from build123d import *

# Parameters (mm, degrees)
BOSS_EXTRUDE1_DEPTH = 5
CUT_EXTRUDE1_DEPTH  = 12
BOSS_EXTRUDE2_DEPTH = 10
FILLET1_R           = 0.5
BOSS_EXTRUDE3_START = -5
SKETCH4_R           = 3.6
BOSS_EXTRUDE3_DEPTH = 6
SKETCH6_R           = 1.6
CUT_EXTRUDE2_DEPTH  = 63.825154198
CUT_EXTRUDE3_DEPTH  = 6


with BuildPart() as part:
    # Sketch1 → Boss-Extrude1 (new body)
    with BuildSketch(Plane(origin=(0, 0, 0), x_dir=(1, 0, 0), z_dir=(0, 1, 0))):
        with BuildLine():
            Line((-44, -35), (44, -35))
            ThreePointArc((44, -35), (48.949747468, -32.949747468), (51, -28))
            Line((51, -28), (51, 28))
            ThreePointArc((51, 28), (48.949747468, 32.949747468), (44, 35))
            Line((44, 35), (-44, 35))
            ThreePointArc((-44, 35), (-48.949747468, 32.949747468), (-51, 28))
            Line((-51, 28), (-51, -28))
            ThreePointArc((-51, -28), (-48.949747468, -32.949747468), (-44, -35))
        make_face()
    extrude(amount=BOSS_EXTRUDE1_DEPTH)

    # Sketch2 → Cut-Extrude1 (cut)
    with BuildSketch(Plane(origin=(0, 5, 0), x_dir=(1, 0, 0), z_dir=(0, 1, 0))):
        with BuildLine():
            Line((-11, -29), (11, -29))
            ThreePointArc((11, -29), (12.5, -30.5), (11, -32))
            Line((11, -32), (-11, -32))
            ThreePointArc((-11, -32), (-12.5, -30.5), (-11, -29))
        make_face()
        with BuildLine():
            Line((-11, 29), (11, 29))
            ThreePointArc((11, 29), (12.5, 30.5), (11, 32))
            Line((11, 32), (-11, 32))
            ThreePointArc((-11, 32), (-12.5, 30.5), (-11, 29))
        make_face()
        with BuildLine():
            Line((-20, 6), (-20, -6))
            ThreePointArc((-20, -6), (-21.5, -7.5), (-23, -6))
            Line((-23, -6), (-23, 6))
            ThreePointArc((-23, 6), (-21.5, 7.5), (-20, 6))
        make_face()
        with BuildLine():
            Line((-10, 6), (-10, -6))
            ThreePointArc((-10, -6), (-11.5, -7.5), (-13, -6))
            Line((-13, -6), (-13, 6))
            ThreePointArc((-13, 6), (-11.5, 7.5), (-10, 6))
        make_face()
        with BuildLine():
            Line((10, 6), (10, -6))
            ThreePointArc((10, -6), (11.5, -7.5), (13, -6))
            Line((13, -6), (13, 6))
            ThreePointArc((13, 6), (11.5, 7.5), (10, 6))
        make_face()
        with BuildLine():
            Line((20, 6), (20, -6))
            ThreePointArc((20, -6), (21.5, -7.5), (23, -6))
            Line((23, -6), (23, 6))
            ThreePointArc((23, 6), (21.5, 7.5), (20, 6))
        make_face()
    extrude(amount=-CUT_EXTRUDE1_DEPTH, mode=Mode.SUBTRACT)

    # Sketch3 → Boss-Extrude2 (add)
    with BuildSketch(Plane(origin=(0, 5, 0), x_dir=(1, 0, 0), z_dir=(0, 1, 0))):
        with BuildLine():
            ThreePointArc((-44.902157539, 17.733333333), (-47, 0), (-44.902157539, -17.733333333))
            ThreePointArc((-44.902157539, -17.733333333), (-43.696427396, -18.47239681), (-42.957363919, -17.266666667))
            ThreePointArc((-42.957363919, -17.266666667), (-45, 0), (-42.957363919, 17.266666667))
            ThreePointArc((-42.957363919, 17.266666667), (-43.696427396, 18.47239681), (-44.902157539, 17.733333333))
        make_face()
        with BuildLine():
            ThreePointArc((43.957363919, 17.266666667), (46, 0), (43.957363919, -17.266666667))
            ThreePointArc((43.957363919, -17.266666667), (44.696427396, -18.47239681), (45.902157539, -17.733333333))
            ThreePointArc((45.902157539, -17.733333333), (48, 0), (45.902157539, 17.733333333))
            ThreePointArc((45.902157539, 17.733333333), (44.696427396, 18.47239681), (43.957363919, 17.266666667))
        make_face()
    extrude(amount=BOSS_EXTRUDE2_DEPTH)

    # Fillet1
    fillet1_edges = [part.edges().sort_by_distance(p)[0] for p in [
        (0, 0, -29),
        (12.5, 0, -30.5),
        (0, 0, -32),
        (-12.5, 0, -30.5),
        (0, 0, 32),
        (12.5, 0, 30.5),
        (0, 0, 29),
        (-12.5, 0, 30.5),
        (-12.5, 5, 30.5),
        (0, 5, 32),
        (12.5, 5, 30.5),
        (0, 5, 29),
        (-12.5, 5, -30.5),
        (0, 5, -29),
        (12.5, 5, -30.5),
        (0, 5, -32),
    ]]
    fillet(fillet1_edges, radius=FILLET1_R)

    # Sketch4 → Boss-Extrude3 (add)
    with BuildSketch(Plane(origin=(0, 5, 0), x_dir=(1, 0, 0), z_dir=(0, 1, 0)).offset(BOSS_EXTRUDE3_START)):
        with Locations(Location((-44, 28, 0), (0, 0, 90))):
            Circle(SKETCH4_R)
        with Locations(Location((-44, -28, 0), (0, 0, 90))):
            Circle(SKETCH4_R)
        with Locations(Location((44, -28, 0), (0, 0, 90))):
            Circle(SKETCH4_R)
        with Locations(Location((44, 28, 0), (0, 0, 90))):
            Circle(SKETCH4_R)
    extrude(amount=-BOSS_EXTRUDE3_DEPTH)

    # Sketch6 → Cut-Extrude2 (cut, through all)
    with BuildSketch(Plane(origin=(0, 5, 0), x_dir=(1, 0, 0), z_dir=(0, 1, 0))):
        with Locations(Location((-44, 28, 0), (0, 0, 270))):
            Circle(SKETCH6_R)
        with Locations(Location((44, 28, 0), (0, 0, 270))):
            Circle(SKETCH6_R)
        with Locations(Location((44, -28, 0), (0, 0, 90))):
            Circle(SKETCH6_R)
        with Locations(Location((-44, -28, 0), (0, 0, 90))):
            Circle(SKETCH6_R)
    extrude(amount=-CUT_EXTRUDE2_DEPTH, mode=Mode.SUBTRACT)

    # Sketch7 → Cut-Extrude3 (cut)
    with BuildSketch(Plane(origin=(0, 5, 0), x_dir=(1, 0, 0), z_dir=(0, 1, 0))):
        Polygon((-42.41228676, 30.75), (-45.58771324, 30.75), (-47.175426481, 28), (-45.58771324, 25.25), (-42.41228676, 25.25), (-40.824573519, 28), align=None)
        Polygon((40.824573519, 28), (42.41228676, 30.75), (45.58771324, 30.75), (47.175426481, 28), (45.58771324, 25.25), (42.41228676, 25.25), align=None)
        Polygon((42.41228676, -30.75), (45.58771324, -30.75), (47.175426481, -28), (45.58771324, -25.25), (42.41228676, -25.25), (40.824573519, -28), align=None)
        Polygon((-40.824573519, -28), (-42.41228676, -30.75), (-45.58771324, -30.75), (-47.175426481, -28), (-45.58771324, -25.25), (-42.41228676, -25.25), align=None)
    extrude(amount=-CUT_EXTRUDE3_DEPTH, mode=Mode.SUBTRACT)


solid = part.part
The listing builds one solid part. Answer for the finished solid, in the listing's coordinates (mm). A direction names the side the tool comes from. Coordinates: 2 decimals unless noted, no trailing zeros. Write each loop counter-clockwise with the first axis right and the second up, starting at its lowest first coordinate (ties: lowest second). Pieces come first, ordered by that corner, then holes. Notation, with made-up numbers: M 61.5,22.25 L 90.5,22.25 A29 ccw 90.5,59.25 Z; hole C 46,14 d5. An arc over 180 degrees is marked long. Put each result on its own line as item: value. Start each with the question number.
1. Which of the six approach directions +Z, -Z, +X, -X, +Y, -Y give full straight-line access (tool end or side, diameter ignored) to faces 1 (the flat face through (-45.4, -1, 29.2)), 2 (the cylindrical face through (21.5, 2.5, 7.5))?
2. For a pull along X with two mould halves and no side action, classify faces 3 (the flat face through (-42.6, -1, -26.8)), 4 (the cylindrical face through (-47, 10, 0)), 5 (the cylindrical face through (48.9, 2.5, 33)), 6 (the flat face through (-23, 3, 0)) as pulls with the +X half, pulls with the -X half, needs draft (parallel to the pull), parting line crosses it, or undercut.
3. Consider line 1 (Z direction, x = -9.5, y = 3.5); line 2 (X direction, y = -3.8, z = -28); line 3 (Y direction, x = -7.5, z = 20). Determine where each line is inside the solid, lowest interval first. Write a range as from..to.
4. A cutting plane is placed at D-D on z = 1. Write down the section's boundary in (x, y), then the cut area to 3 significant figures.
5. A cutting plane is placed at C-C on x = -5. Write down the section's boundary in (y, z).
6. A cutting plane is placed at A-A on x = -21.5. Write down the section's boundary in (y, z), then the cut area to 3 significant figures.
7. A cutting plane is placed at B-B on y = 8.25. Write down the section's boundary in (x, z).
8. Flat-ended cylindrical pins translate along their axes: P1, Ø1, axis at x = 44.5, y = 0.5, coming from the -Z side; P2, Ø8, axis at x = 22.5, z = -12, coming from the +Y side; P3, Ø5, axis at y = 11.5, z = 19.5, coming from the -X side; P4, Ø4, axis at x = -11.5, z = 15, coming from the -Y side. Find the tip coordinate at first contact, or state that the pin passes through.
Resolved:
1. face 1: +Y
1. face 2: +Y, -Y
2. face 3: undercut
2. face 4: pulls with the -X half
2. face 5: pulls with the +X half
2. face 6: undercut
3. line 1: z = -35..-32, -29..29, 32..35
3. line 2: x = -47.6..-45.6, -42.4..-40.4, 40.4..42.4, 45.6..47.6
3. line 3: y = 0..5
4. outline: M -51,0 L -23,0 L -23,5 L -44.99,5 L -44.99,15 L -46.99,15 L -46.99,5 L -51,5 Z; M -20,0 L -13,0 L -13,5 L -20,5 Z; M -10,0 L 10,0 L 10,5 L -10,5 Z; M 13,0 L 20,0 L 20,5 L 13,5 Z; M 23,0 L 51,0 L 51,5 L 47.99,5 L 47.99,15 L 45.99,15 L 45.99,5 L 23,5 Z
4. area: 490 mm2
5. outline: M 0,-35 L 5,-35 L 5,-32.5 A0.5 ccw 4.5,-32 L 0.5,-32 A0.5 ccw 0,-32.5 Z; M 0,-28.5 A0.5 ccw 0.5,-29 L 4.5,-29 A0.5 ccw 5,-28.5 L 5,28.5 A0.5 ccw 4.5,29 L 0.5,29 A0.5 ccw 0,28.5 Z; M 0,32.5 A0.5 ccw 0.5,32 L 4.5,32 A0.5 ccw 5,32.5 L 5,35 L 0,35 Z
6. outline: M 0,-35 L 5,-35 L 5,-7.5 L 0,-7.5 Z; M 0,7.5 L 5,7.5 L 5,35 L 0,35 Z
6. area: 275 mm2
7. outline: M -44.9,-17.73 A1 ccw -42.96,-17.27 A74 cw -42.96,17.27 A1 ccw -44.9,17.73 A76 ccw Z; M 43.96,-17.27 A1 ccw 45.9,-17.73 A76 ccw 45.9,17.73 A1 ccw 43.96,17.27 A74 cw Z
8. P1: stops at z = -35
8. P2: stops at y = 5
8. P3: stops at x = -45.07
8. P4: stops at y = 0
